Part model, mm, in its own coordinate system. Face numbers are marked on the shaded views. Give positions to 0.01 mm unless a question says otherwise; leave off trailing zeros. Order: outer loops, then holes, each group sorted by start corner. A loop starts at its lowest first (then second) coordinate and runs counter-clockwise, first axis right, second up. Notation, with made-up numbers: (18.5, 62.25) -> (32.5, 62.25) arc R33 ccw to (32.5, 98.25) -> close; hole circle Ø5 at (2, 43). An arc over 180 degrees is marked (long way). Write item = value, one per line. Start each with the question number.
(1) Saw through at A-A, the plane y = 10.75. List the corners of the cut face in (x, z).
(2) Probe line 1 along Z through (x, y) = (0, 7.25); line 2 along Y through (x, z) = (2, 4.5); line 3 along Y through (x, z) = (3.75, 2.5). List the from-to ranges inside material, lowest first. Write a range as from..to.
(3) Saw through at B-B, the plane y = 14.25. List the corners of the cut face in (x, z), then the cut area to 3 significant figures.
(4) Two-plate mould, pull along X, no slides. Class the marked faces 1, 2 and 3: pulls with the +X half, pulls with the -X half, needs draft (parallel to the pull), parting line crosses it, or undercut.
(5) Flat gauge pins, fed straight in: pin 1 (4 mm diameter, centred on x = -1.5, y = 9.5, fed in from -Z); pin 2 (1.5 mm diameter, centred on y = 11.5, z = 4.5, fed in from +X); pin 3 (8 mm diameter, centred on x = 7.5, z = -5.5, fed in from -Y); pin 4 (1.5 mm diameter, centred on x = -3.5, y = 6.5, fed in from +Z). Where does each tip first touch, or does it go through?
from build123d import *

# Parameters (mm, degrees)
KES_EKSTR_ZYON1_REACH = 25.956
IZIM2_R               = 2.5
KES_S_P_R1_PITCH      = 1.25
KES_S_P_R1_TO         = 5


with BuildPart() as part:
    # Çizim1 → Döndür1 (revolve)
    with BuildSketch(Plane.XY, mode=Mode.PRIVATE) as d_nd_r1_sk:
        with BuildLine():
            Line((0, -1.027887155), (5, -1.027887155))
            Line((5, -1.027887155), (5, 3.972112845))
            Line((5, 3.972112845), (8.32455532, 3.972112845))
            ThreePointArc((8.32455532, 3.972112845), (9.031662102, 4.265006064), (9.32455532, 4.972112845))
            Line((9.32455532, 4.972112845), (9.32455532, 11.034858912))
            ThreePointArc((9.32455532, 11.034858912), (9.07455532, 11.69629674), (8.44955532, 12.027015654))
            ThreePointArc((8.44955532, 12.027015654), (5.322926591, 13.228684643), (3.112574113, 15.745459861))
            ThreePointArc((3.112574113, 15.745459861), (3.028551111, 15.969161353), (3, 16.206410287))
            Line((3, 16.206410287), (3, 18.472112845))
            ThreePointArc((3, 18.472112845), (2.853553391, 18.825666236), (2.5, 18.972112845))
            Line((2.5, 18.972112845), (0, 18.972112845))
            Line((0, 18.972112845), (0, 15.972112845))
            Line((0, 15.972112845), (0, -1.027887155))
        make_face()
    revolve(d_nd_r1_sk.sketch.rotate(Axis((0, 15.972112845, 0), (0, -1, 0)), 180), axis=Axis((0, 15.972112845, 0), (0, -1, 0)))

    # Çizim2 → Kes-Ekstrüzyon1 (cut, up to next)
    with BuildSketch(Plane(origin=(0, 18.972112845, 0), x_dir=(1, 0, 0), z_dir=(0, 1, 0)), mode=Mode.PRIVATE) as kes_ekstr_zyon1_sk1:
        with Locations(Location((0, 0, 0), (0, 0, 180))):
            Circle(IZIM2_R)
    kes_ekstr_zyon1_tool1 = extrude(kes_ekstr_zyon1_sk1.sketch, amount=-KES_EKSTR_ZYON1_REACH, mode=Mode.PRIVATE) & part.part
    add(kes_ekstr_zyon1_tool1.solids().sort_by_distance((0, 18.972113, 0))[0], mode=Mode.SUBTRACT)

    # Kes-Süpür1: arcs per turn and ends read off the stored shape
    # Kes-Süpür1: the profile of Çizim7 screwed along a right-hand helix through 5.5 turns, 8 arcs to a turn; built about Z, then put on its axis
    kes_s_p_r1_z = Axis((0, 0, 0), (0, 0, 1))
    kes_s_p_r1_corners = [(4.250843742, 0, -1.25), (5.085388022, 0, -0.551697778), (5.085388022, 0, -1.25)]
    with BuildLine(mode=Mode.PRIVATE) as kes_s_p_r1_profile:
        Line(kes_s_p_r1_corners[0], kes_s_p_r1_corners[1])
        Line(kes_s_p_r1_corners[1], kes_s_p_r1_corners[2])
        Line(kes_s_p_r1_corners[2], kes_s_p_r1_corners[0])
    kes_s_p_r1_cap = Face(kes_s_p_r1_profile.wire())
    kes_s_p_r1_turn_angles = [0, 22.5, 45, 67.5, 90, 112.5, 135, 157.5, 180, 202.5, 225, 247.5, 270, 292.5, 315, 337.5, 360]
    kes_s_p_r1_turn_weights = [1, 0.9238795325112867, 1, 0.9238795325112867, 1, 0.9238795325112867, 1, 0.9238795325112867, 1, 0.9238795325112867, 1, 0.9238795325112867, 1, 0.9238795325112867, 1, 0.9238795325112867, 1]
    kes_s_p_r1_turn_rails = [Edge.make_bspline([Vector(p[0], p[1], 0).rotate(kes_s_p_r1_z, kes_s_p_r1_turn_angles[k]) / kes_s_p_r1_turn_weights[k] + Vector(0, 0, p[2] + KES_S_P_R1_PITCH * kes_s_p_r1_turn_angles[k] / 360) for k in range(17)], [0, 0, 0, 1, 1, 2, 2, 3, 3, 4, 4, 5, 5, 6, 6, 7, 7, 8, 8, 8], 2, kes_s_p_r1_turn_weights) for p in kes_s_p_r1_corners]
    kes_s_p_r1_turn_sides = [Face.make_surface_from_curves(kes_s_p_r1_turn_rails[p[0]], kes_s_p_r1_turn_rails[p[1]]) for p in [(0, 1), (1, 2), (2, 0)]]
    kes_s_p_r1_last_angles = [1800, 1822.5, 1845, 1867.5, 1890, 1912.5, 1935, 1957.5, 1980]
    kes_s_p_r1_last_weights = [1, 0.9238795325112867, 1, 0.9238795325112867, 1, 0.9238795325112867, 1, 0.9238795325112867, 1]
    kes_s_p_r1_last_rails = [Edge.make_bspline([Vector(p[0], p[1], 0).rotate(kes_s_p_r1_z, kes_s_p_r1_last_angles[k]) / kes_s_p_r1_last_weights[k] + Vector(0, 0, p[2] + KES_S_P_R1_PITCH * kes_s_p_r1_last_angles[k] / 360) for k in range(9)], [0, 0, 0, 1, 1, 2, 2, 3, 3, 4, 4, 4], 2, kes_s_p_r1_last_weights) for p in kes_s_p_r1_corners]
    kes_s_p_r1_last_sides = [Face.make_surface_from_curves(kes_s_p_r1_last_rails[p[0]], kes_s_p_r1_last_rails[p[1]]) for p in [(0, 1), (1, 2), (2, 0)]]
    kes_s_p_r1 = Plane(origin=(0, -1.027887155, 0), x_dir=(-1, 0, 0), z_dir=(0, 1, 0)) * split(Solid(Shell([*[p.moved(Location((0, 0, KES_S_P_R1_PITCH * i))) for i in range(5) for p in kes_s_p_r1_turn_sides], *kes_s_p_r1_last_sides, kes_s_p_r1_cap, kes_s_p_r1_cap.rotate(kes_s_p_r1_z, 1980).moved(Location((0, 0, KES_S_P_R1_PITCH * 1980 / 360)))])), bisect_by=Plane.XY.offset(KES_S_P_R1_TO), keep=Keep.BOTTOM, mode=Mode.PRIVATE)
    add(kes_s_p_r1, mode=Mode.SUBTRACT)


solid = part.part
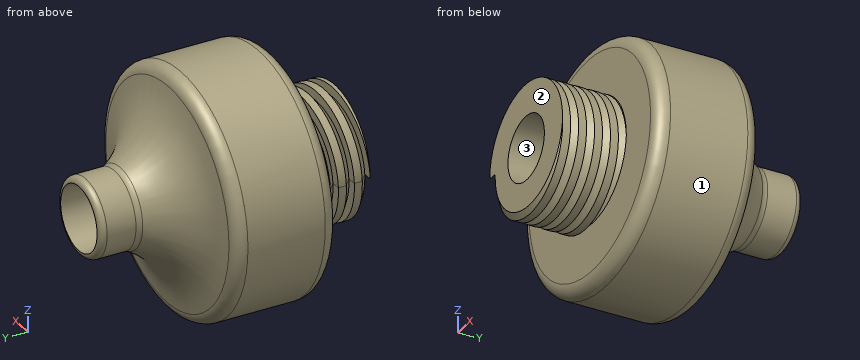
Results list:
q1.outline = circle Ø18.65 at (0, 0); hole circle Ø5 at (0, 0)
q2.line_1 = -9.32..-2.5, 2.5..9.32
q2.line_2 = -1.03..-0.63, -0.07..0.62, 1.18..1.87, 2.43..3.12, 3.68..13.53
q2.line_3 = -1.03..-0.52, -0.31..0.73, 0.94..1.98, 2.19..3.23, 3.44..13.89
q3.outline = circle Ø8.31 at (0, 0); hole circle Ø5 at (0, 0)
q3.area = 34.7 mm^2
q4.face_1 = parting line crosses it
q4.face_2 = needs draft
q4.face_3 = undercut
q5.pin_1 = -9.32
q5.pin_2 = 8.49
q5.pin_3 = 3.97
q5.pin_4 = 8.91
